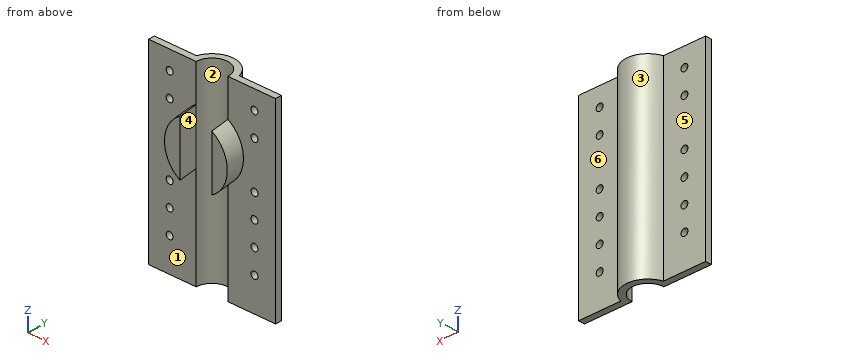
from build123d import *

# Parameters (mm, degrees)
BOSS_EXTRUDE1_DEPTH      = 100
BOSS_EXTRUDE1_DEPTH_BACK = 50
CUT_EXTRUDE2_REACH       = 115.345
SKETCH6_R                = 2.7


with BuildPart() as part:
    # Sketch1 → Boss-Extrude1 (new, two sides: drawn at the far end of the back side and taken through both)
    with BuildSketch(Plane.XY.offset(-BOSS_EXTRUDE1_DEPTH_BACK)):
        with BuildLine():
            Line((-12.5, 0), (-50, 0))
            Line((-50, 0), (-50, 5))
            Line((-50, 5), (-16.770509831, 5))
            ThreePointArc((-16.770509831, 5), (0, 17.5), (16.770509831, 5))
            Line((16.770509831, 5), (50, 5))
            Line((50, 5), (50, 0))
            Line((50, 0), (12.5, 0))
            ThreePointArc((12.5, 0), (0, 12.5), (-12.5, 0))
        make_face()
    extrude(amount=BOSS_EXTRUDE1_DEPTH + BOSS_EXTRUDE1_DEPTH_BACK)

    # Sweep1: sweep along a path in Sketch4
    with BuildLine(Plane.ZY.offset(12.5)) as sweep1_path:
        Line((50.0437673, 0), (48.0549131, -13.633099982))
    # Sketch3 → Sweep1 (sweep)
    with BuildSketch(Plane.XZ):
        with BuildLine():
            Line((-12.5, 71.352170208), (-12.5, 28.735364392))
            ThreePointArc((-12.5, 28.735364392), (-24.704210866, 50.0437673), (-12.5, 71.352170208))
        make_face()
        with BuildLine():
            Line((12.5, 71.352170208), (12.5, 28.735364392))
            ThreePointArc((12.5, 28.735364392), (24.704210866, 50.0437673), (12.5, 71.352170208))
        make_face()
    sweep(path=sweep1_path.line)

    # Sketch6 → Cut-Extrude2 (cut, up to next)
    with BuildSketch(Plane(origin=(0, 5, 0), x_dir=(1, 0, 0), z_dir=(0, 1, 0)), mode=Mode.PRIVATE) as cut_extrude2_sk1:
        with Locations(Location((-33.385254916, 24.07, 0), (0, 0, 180))):
            Circle(SKETCH6_R)
    cut_extrude2_tool1 = extrude(cut_extrude2_sk1.sketch, amount=-CUT_EXTRUDE2_REACH, mode=Mode.PRIVATE) & part.part
    # Sketch6 → Cut-Extrude2 (cut, up to next)
    with BuildSketch(Plane(origin=(0, 5, 0), x_dir=(1, 0, 0), z_dir=(0, 1, 0)), mode=Mode.PRIVATE) as cut_extrude2_sk2:
        with Locations(Location((-33.385254916, 5.67, 0), (0, 0, 180))):
            Circle(SKETCH6_R)
    cut_extrude2_tool2 = extrude(cut_extrude2_sk2.sketch, amount=-CUT_EXTRUDE2_REACH, mode=Mode.PRIVATE) & part.part
    # Sketch6 → Cut-Extrude2 (cut, up to next)
    with BuildSketch(Plane(origin=(0, 5, 0), x_dir=(1, 0, 0), z_dir=(0, 1, 0)), mode=Mode.PRIVATE) as cut_extrude2_sk3:
        with Locations(Location((-33.385254916, -12.73, 0), (0, 0, 180))):
            Circle(SKETCH6_R)
    cut_extrude2_tool3 = extrude(cut_extrude2_sk3.sketch, amount=-CUT_EXTRUDE2_REACH, mode=Mode.PRIVATE) & part.part
    # Sketch6 → Cut-Extrude2 (cut, up to next)
    with BuildSketch(Plane(origin=(0, 5, 0), x_dir=(1, 0, 0), z_dir=(0, 1, 0)), mode=Mode.PRIVATE) as cut_extrude2_sk4:
        with Locations(Location((-33.385254916, -31.13, 0), (0, 0, 180))):
            Circle(SKETCH6_R)
    cut_extrude2_tool4 = extrude(cut_extrude2_sk4.sketch, amount=-CUT_EXTRUDE2_REACH, mode=Mode.PRIVATE) & part.part
    # Sketch6 → Cut-Extrude2 (cut, up to next)
    with BuildSketch(Plane(origin=(0, 5, 0), x_dir=(1, 0, 0), z_dir=(0, 1, 0)), mode=Mode.PRIVATE) as cut_extrude2_sk5:
        with Locations(Location((-33.385254916, -67.13, 0), (0, 0, 180))):
            Circle(SKETCH6_R)
    cut_extrude2_tool5 = extrude(cut_extrude2_sk5.sketch, amount=-CUT_EXTRUDE2_REACH, mode=Mode.PRIVATE) & part.part
    # Sketch6 → Cut-Extrude2 (cut, up to next)
    with BuildSketch(Plane(origin=(0, 5, 0), x_dir=(1, 0, 0), z_dir=(0, 1, 0)), mode=Mode.PRIVATE) as cut_extrude2_sk6:
        with Locations(Location((-33.385254916, -85.53, 0), (0, 0, 180))):
            Circle(SKETCH6_R)
    cut_extrude2_tool6 = extrude(cut_extrude2_sk6.sketch, amount=-CUT_EXTRUDE2_REACH, mode=Mode.PRIVATE) & part.part
    # Sketch6 → Cut-Extrude2 (cut, up to next)
    with BuildSketch(Plane(origin=(0, 5, 0), x_dir=(1, 0, 0), z_dir=(0, 1, 0)), mode=Mode.PRIVATE) as cut_extrude2_sk7:
        with Locations(Location((33.385254916, 24.07, 0), (0, 0, 180))):
            Circle(SKETCH6_R)
    cut_extrude2_tool7 = extrude(cut_extrude2_sk7.sketch, amount=-CUT_EXTRUDE2_REACH, mode=Mode.PRIVATE) & part.part
    # Sketch6 → Cut-Extrude2 (cut, up to next)
    with BuildSketch(Plane(origin=(0, 5, 0), x_dir=(1, 0, 0), z_dir=(0, 1, 0)), mode=Mode.PRIVATE) as cut_extrude2_sk8:
        with Locations(Location((33.385254916, 5.67, 0), (0, 0, 180))):
            Circle(SKETCH6_R)
    cut_extrude2_tool8 = extrude(cut_extrude2_sk8.sketch, amount=-CUT_EXTRUDE2_REACH, mode=Mode.PRIVATE) & part.part
    # Sketch6 → Cut-Extrude2 (cut, up to next)
    with BuildSketch(Plane(origin=(0, 5, 0), x_dir=(1, 0, 0), z_dir=(0, 1, 0)), mode=Mode.PRIVATE) as cut_extrude2_sk9:
        with Locations(Location((33.385254916, -31.13, 0), (0, 0, 180))):
            Circle(SKETCH6_R)
    cut_extrude2_tool9 = extrude(cut_extrude2_sk9.sketch, amount=-CUT_EXTRUDE2_REACH, mode=Mode.PRIVATE) & part.part
    # Sketch6 → Cut-Extrude2 (cut, up to next)
    with BuildSketch(Plane(origin=(0, 5, 0), x_dir=(1, 0, 0), z_dir=(0, 1, 0)), mode=Mode.PRIVATE) as cut_extrude2_sk10:
        with Locations(Location((33.385254916, -67.13, 0), (0, 0, 180))):
            Circle(SKETCH6_R)
    cut_extrude2_tool10 = extrude(cut_extrude2_sk10.sketch, amount=-CUT_EXTRUDE2_REACH, mode=Mode.PRIVATE) & part.part
    # Sketch6 → Cut-Extrude2 (cut, up to next)
    with BuildSketch(Plane(origin=(0, 5, 0), x_dir=(1, 0, 0), z_dir=(0, 1, 0)), mode=Mode.PRIVATE) as cut_extrude2_sk11:
        with Locations(Location((33.385254916, -85.53, 0), (0, 0, 180))):
            Circle(SKETCH6_R)
    cut_extrude2_tool11 = extrude(cut_extrude2_sk11.sketch, amount=-CUT_EXTRUDE2_REACH, mode=Mode.PRIVATE) & part.part
    # Sketch6 → Cut-Extrude2 (cut, up to next)
    with BuildSketch(Plane(origin=(0, 5, 0), x_dir=(1, 0, 0), z_dir=(0, 1, 0)), mode=Mode.PRIVATE) as cut_extrude2_sk12:
        with Locations(Location((33.385254916, -12.73, 0), (0, 0, 180))):
            Circle(SKETCH6_R)
    cut_extrude2_tool12 = extrude(cut_extrude2_sk12.sketch, amount=-CUT_EXTRUDE2_REACH, mode=Mode.PRIVATE) & part.part
    add(cut_extrude2_tool1.solids().sort_by_distance((-33.385255, 5, -24.07))[0], mode=Mode.SUBTRACT)
    add(cut_extrude2_tool2.solids().sort_by_distance((-33.385255, 5, -5.67))[0], mode=Mode.SUBTRACT)
    add(cut_extrude2_tool3.solids().sort_by_distance((-33.385255, 5, 12.73))[0], mode=Mode.SUBTRACT)
    add(cut_extrude2_tool4.solids().sort_by_distance((-33.385255, 5, 31.13))[0], mode=Mode.SUBTRACT)
    add(cut_extrude2_tool5.solids().sort_by_distance((-33.385255, 5, 67.13))[0], mode=Mode.SUBTRACT)
    add(cut_extrude2_tool6.solids().sort_by_distance((-33.385255, 5, 85.53))[0], mode=Mode.SUBTRACT)
    add(cut_extrude2_tool7.solids().sort_by_distance((33.385255, 5, -24.07))[0], mode=Mode.SUBTRACT)
    add(cut_extrude2_tool8.solids().sort_by_distance((33.385255, 5, -5.67))[0], mode=Mode.SUBTRACT)
    add(cut_extrude2_tool9.solids().sort_by_distance((33.385255, 5, 31.13))[0], mode=Mode.SUBTRACT)
    add(cut_extrude2_tool10.solids().sort_by_distance((33.385255, 5, 67.13))[0], mode=Mode.SUBTRACT)
    add(cut_extrude2_tool11.solids().sort_by_distance((33.385255, 5, 85.53))[0], mode=Mode.SUBTRACT)
    add(cut_extrude2_tool12.solids().sort_by_distance((33.385255, 5, 12.73))[0], mode=Mode.SUBTRACT)


solid = part.part
Could you check a few things on this model? Use its own coordinates, in mm. Face numbers are marked on the shaded views. A direction names the side the tool comes from. Round coordinates to 2 decimals unless told otherwise and drop trailing zeros. Loops run counter-clockwise (first coordinate to the right, second up) from the corner with the lowest first, then second, coordinate; pieces in that order, holes last. Notation, with made-up numbers: (69.25, -35.75) -> (123.25, -35.75) arc R25 ccw to (123.25, 1.25) -> close; hole circle Ø3 at (-7, 79). An arc over 180 degrees is marked (long way). Use CSV: the item, a comma, the result in double quotes.
(1) Suppose I cut it at C-C on x = 0. Write out the boundary of the cut face in (y, z).
Return value:
outline,"(12.5, -50) -> (17.5, -50) -> (17.5, 100) -> (12.5, 100) -> close"
(2) Will these pins go through, and if not, where does the flat tip stop? pin 1 Ø1 at (x, y) = (-18, -10) entering from -Z; pin 2 Ø7 at (x, z) = (33.39, -24.07) entering from +Y; pin 3 Ø19 at (x, z) = (-33, -9) entering from -Y.
Return value:
pin 1,"stops at z = 31.14"
pin 2,"stops at y = 5"
pin 3,"stops at y = 0"
(3) Suppose I cut it at B-B on y = 6.5. Write out the boundary of the cut face in (x, z), plus the area to 3 significant figures.
Return value:
outline,"(-16.25, -50) -> (-10.68, -50) -> (-10.68, 100) -> (-16.25, 100) -> close; (10.68, -50) -> (16.25, -50) -> (16.25, 100) -> (10.68, 100) -> close"
area,"1,670 mm²"
(4) If we mould it in two halves opening along X, with no side actions, what happens to the marked faces 1, 2, 3 and 4? For each: +X half, -X half, draft (parallel to the pull), parting line (faces both ways), or undercut.
Return value:
face 1,"draft"
face 2,"undercut"
face 3,"parting line"
face 4,"undercut"
(5) For the marked faces 5 and 6, which set-ups out of +Z, -Z, +X, -X, +Y, -Y let a thin tool reach every point of the face, with its end or its side?
Return value:
face 5,"+Z, -Z, -X, +Y"
face 6,"+Z, -Z, +X, +Y"
(6) If I drill on probe 1 along X at (y, z) = (4, 12); probe 2 along Y at (x, z) = (18.5, 8); probe 3 along X at (y, z) = (1, 42.5), over which ranges is the centre line in solid material (lowest first)? Write a range as [from, to].
Return value:
probe 1,"x = [-50, -35.98], [-30.79, -11.84], [11.84, 30.79], [35.98, 50]"
probe 2,"y = [0, 5]"
probe 3,"x = [-50, -12.46], [12.46, 50]"
(7) Suppose I cut it at A-A on z = 12.73. Write out the boundary of the cut face in (x, y), plus the area to 3 significant figures.
Return value:
outline,"(-50, 0) -> (-36.09, 0) -> (-36.09, 5) -> (-50, 5) -> close; (-30.69, 0) -> (-12.5, 0) arc R12.5 cw to (12.5, 0) -> (30.69, 0) -> (30.69, 5) -> (16.77, 5) arc R17.5 ccw to (-16.77, 5) -> (-30.69, 5) -> close; (36.09, 0) -> (50, 0) -> (50, 5) -> (36.09, 5) -> close"
area,"509 mm²"
(8) Suppose I cut it at D-D on z = 31.13. Give the number of separate pieces and of enclosed holes in the cut face, plus the area to 3 significant figures.
Return value:
separate pieces,"3"
enclosed holes,"0"
area,"631 mm²"
